Part model, mm, in its own coordinate system. Face numbers are marked on the shaded views. Give positions to 0.01 mm unless a question says otherwise; leave off trailing zeros. Write each loop counter-clockwise with the first axis right and the second up, starting at its lowest first coordinate (ties: lowest second). Pieces come first, ordered by that corner, then holes. Notation, with made-up numbers: M 14.25,-38 L 24.25,-38 A16 ccw 24.25,-17 Z; hole C 24,-27.5 d9. An arc over 180 degrees is marked long. Use a Markdown table: item, result. Add a question column.
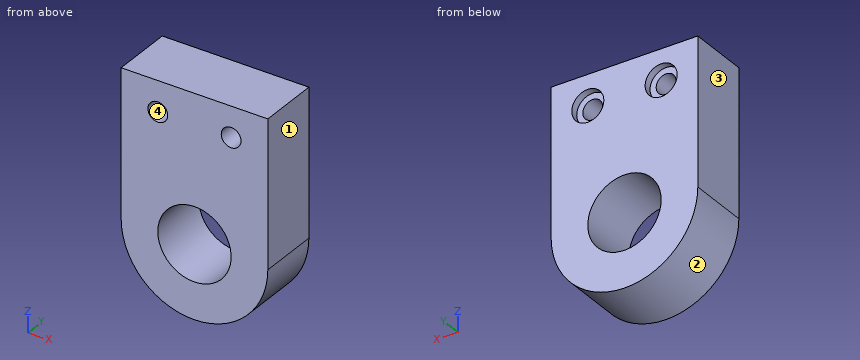
Autodesk Inventor part; units mm, degrees
ref_plane "YZ Plane" through (0, 0, 0) normal (1, 0, 0) x (0, 1, 0)
ref_plane "XZ Plane" through (0, 0, 0) normal (0, 1, 0) x (-1, 0, 0)
ref_plane "XY Plane" through (0, 0, 0) normal (0, 0, 1) x (1, 0, 0)
sketch "Sketch1" plane through (0, 0, 0) normal (0, 1, 0) x (-1, 0, 0)
  line L0 (30, 60) -> (-30, 60)
  line L1 (-30, 60) -> (-30, 0)
  arc A0 (-30, 0) -> (30, 0) centre (0, 0) ccw
  line L2 (30, 0) -> (30, 60)
  circle A1 centre (0, 0) radius 15
  dimension "d0" = 60
  dimension "d1" = 60
  dimension "d2" = 30
extrude "Extrusion1" add sketch "Sketch1" along normal mid plane 25
sketch "Sketch2" plane through (0, 0, 0) normal (0, 1, 0) x (-1, 0, 0)
  line L0 (-30, 0) -> (-30, 60) construction
  line L1 (-30, 60) -> (30, 60) construction
  line L2 (30, 60) -> (30, 0) construction
  arc A0 (-30, 0) -> (30, 0) centre (0, 0) ccw construction
  circle A1 centre (0, 0) radius 15 construction
  line L3 (30, 60) -> (30, 0) construction
  line L4 (30, 35) -> (-30, 35) construction
  circle A2 centre (15, 47.5) radius 4.05
  line L5 (0, 35) -> (0, 60) construction
  circle A3 centre (-15, 47.5) radius 4.05
  point P0 (0, -30)
  point P1 (0, 47.5)
  dimension "d5" = 65
  dimension "d6" = 8.1
  dimension "d7" = 30
extrude "Extrusion2" cut sketch "Sketch2" along normal through all both and the other way through all
sketch "Sketch3" plane through (0, 12.5, 0) normal (0, 1, 0) x (1, 0, 0)
  circle A0 centre (-15, -47.5) radius 4.05 construction
  circle A1 centre (15, -47.5) radius 4.05 construction
  line L0 (30, -60) -> (30, 0) construction
  arc A2 (30, 0) -> (-30, 0) centre (0, 0) ccw construction
  line L1 (-30, 0) -> (-30, -60) construction
  line L2 (-30, -60) -> (30, -60) construction
  circle A3 centre (0, 0) radius 15 construction
  circle A4 centre (-15, -47.5) radius 4.05
  circle A5 centre (-15, -47.5) radius 6.55
  circle A6 centre (15, -47.5) radius 6.55
  dimension "d10" = 13.1
  dimension "d11" = 13.1
extrude "Extrusion3" cut sketch "Sketch3" against normal blind 3 contours A4 | A5 | A6
properties part number "element3_obj4"
1. Cut at D-D (x = -13.5). Write the cut outline in (y, z).
2. Drill centre lines: probe 1 along X at (y, z) = (-0.75, 47.5); probe 2 along X at (y, z) = (10.1, 47.5); probe 3 along Z at (x, y) = (5, -5.5). Where is each one in solid material? Low to high. Write a range as [from, to].
3. Flat gauge pins, fed straight in: pin 1 (13 mm diameter, centred on x = -15, z = 47.5, fed in from +Y); pin 2 (8 mm diameter, centred on x = 15, z = 47.5, fed in from -Y); pin 3 (4 mm diameter, centred on y = 8.5, z = -9, fed in from +X); pin 4 (2 mm diameter, centred on y = 6.5, z = -11.5, fed in from -X). Where does each tip first touch, or does it go through?
4. Mould opens along X. For the marked faces 1, 2, 3 and 4 say: released by +X, released by -X, zero draft, split by the parting line, or undercut.
5. Cut at C-C (z = 47.5). Write the cut outline in (x, y).
6. Cut at B-B (x = 0). Write the cut outline in (y, z).
7. Cut at A-A (y = -10.25). Write the cut outline in (x, z).
A:
| question | item | result |
|---|---|---|
| 1 | outline | M -12.5,-26.79 L 12.5,-26.79 L 12.5,-6.54 L -12.5,-6.54 Z; M -12.5,6.54 L 12.5,6.54 L 12.5,41.12 L 9.5,41.12 L 9.5,43.74 L -12.5,43.74 Z; M -12.5,51.26 L 9.5,51.26 L 9.5,53.88 L 12.5,53.88 L 12.5,60 L -12.5,60 Z |
| 2 | probe 1 | x = [-30, -19.05], [-10.95, 10.95], [19.05, 30] |
| 2 | probe 2 | x = [-30, -21.55], [-8.45, 8.45], [21.55, 30] |
| 2 | probe 3 | z = [-29.58, -14.14], [14.14, 60] |
| 3 | pin 1 | stops at y = 9.5 |
| 3 | pin 2 | passes through |
| 3 | pin 3 | stops at x = 29.17 |
| 3 | pin 4 | stops at x = -28.1 |
| 4 | face 1 | released by +X |
| 4 | face 2 | split by the parting line |
| 4 | face 3 | released by -X |
| 4 | face 4 | undercut |
| 5 | outline | M -30,-12.5 L -19.05,-12.5 L -19.05,9.5 L -21.55,9.5 L -21.55,12.5 L -30,12.5 Z; M -10.95,-12.5 L 10.95,-12.5 L 10.95,9.5 L 8.45,9.5 L 8.45,12.5 L -8.45,12.5 L -8.45,9.5 L -10.95,9.5 Z; M 19.05,-12.5 L 30,-12.5 L 30,12.5 L 21.55,12.5 L 21.55,9.5 L 19.05,9.5 Z |
| 6 | outline | M -12.5,-30 L 12.5,-30 L 12.5,-15 L -12.5,-15 Z; M -12.5,15 L 12.5,15 L 12.5,60 L -12.5,60 Z |
| 7 | outline | M -30,0 A30 ccw 30,0 L 30,60 L -30,60 Z; hole C -15,47.5 d8.1; hole C 0,0 d30; hole C 15,47.5 d8.1 |
